Check sheet for the modelled part. Datum: model origin and axes. Units: mm. Face numbers are marked on the shaded views. A direction names the side the tool comes from. Round coordinates to 2 decimals unless told otherwise and drop trailing zeros. Loops run counter-clockwise (first coordinate to the right, second up) from the corner with the lowest first, then second, coordinate; pieces in that order, holes last. Notation, with made-up numbers: (-6, 12) -> (36, 12) arc R31 cw to (36, 46) -> close; hole circle Ø5 at (6.5, -13). An arc over 180 degrees is marked (long way). One line per question, with ' | ' between items.
```python
from build123d import *

# Parameters (mm, degrees)
F1_DEPTH = 5
F2_W     = 5
F2_H     = 5
F3_DEPTH = 12
F4_R     = 1.5
F5_DEPTH = 20


with BuildPart() as f1:
    # F0 (on Right) → F1 (new body, symmetric)
    with BuildSketch(Plane.YZ):
        Polygon((-5.680779, 3.206832), (-10.680779, 3.206832), (-20.680779, -6.793168), (-5.680779, -6.793168), align=None)
    extrude(amount=F1_DEPTH, both=True)

    # F2 (on face) → F3 (join)
    with BuildSketch(Plane.XY.offset(3.206832)):
        with Locations((2.5, -8.180779)):
            Rectangle(F2_W, F2_H)
    extrude(amount=F3_DEPTH)

    # F4 (on face) → F5 (join)
    with BuildSketch(Plane.XY.offset(3.206832)):
        with Locations((-2.5, -8.180779)):
            Circle(F4_R)
    extrude(amount=F5_DEPTH)


solid = f1.part
```
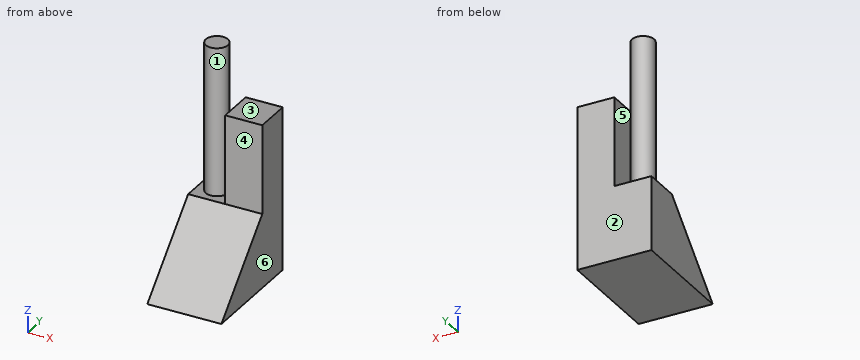
(1) Sectioned sample at A-A, the plane x = -2.75. Record the cut outline in (y, z).
Answer:
outline: (-20.68, -6.79) -> (-5.68, -6.79) -> (-5.68, 3.21) -> (-6.7, 3.21) -> (-6.7, 23.21) -> (-9.66, 23.21) -> (-9.66, 3.21) -> (-10.68, 3.21) -> close
(2) Go/stop test with flat-tipped pins: pin 1 (5.5 mm diameter, centred on x = 1.5, y = -7.5, fed in from +Z); pin 2 (1 mm diameter, centred on x = -2, y = -17, fed in from +Z); pin 3 (1.5 mm diameter, centred on x = 1.5, z = 7.5, fed in from -Y); pin 4 (6 mm diameter, centred on y = -12, z = 13, fed in from -X). Record where each tip stops, or that it passes through.
Answer:
pin 1: stops at z = 23.21 | pin 2: stops at z = -2.61 | pin 3: stops at y = -10.68 | pin 4: stops at x = -3.76
(3) Sectioned sample at D-D, the plane z = -1.5. Record the cut outline in (x, y), and give its area (3 significant figures).
Answer:
outline: (-5, -15.39) -> (5, -15.39) -> (5, -5.68) -> (-5, -5.68) -> close | area: 97.1 mm2
(4) Mould release check, pull along X, two halves, no side actions. Record for the marked faces 4, 5 and 6: +X half, -X half, draft (parallel to the pull), parting line (faces both ways), or undercut.
Answer:
face 4: draft | face 5: undercut | face 6: +X half
(5) Set-up check for the marked faces 1, 2 and 3: record each of +Z, -Z, +X, -X, +Y, -Y from which the full face is reachable in a straight line by a thin tool's end or side.
Answer:
face 1: +Z | face 2: +Z, -Z, +X, -X, +Y | face 3: +Z, +X, +Y, -Y
(6) Sectioned sample at B-B, the plane z = 7. Record the cut outline in (x, y), and give its area (3 significant figures).
Answer:
outline: circle Ø3 at (-2.5, -8.18); (0, -10.68) -> (5, -10.68) -> (5, -5.68) -> (0, -5.68) -> close | area: 32.1 mm2
(7) Sectioned sample at C-C, the plane y = -7.5. Record the cut outline in (x, z).
Answer:
outline: (-5, -6.79) -> (5, -6.79) -> (5, 15.21) -> (0, 15.21) -> (0, 3.21) -> (-1.16, 3.21) -> (-1.16, 23.21) -> (-3.84, 23.21) -> (-3.84, 3.21) -> (-5, 3.21) -> close
(8) Scan lines: probe 1 along Y at (x, z) = (-2.5, 7.25); probe 2 along Z at (x, y) = (2.25, -8); probe 3 along X at (y, z) = (-10.5, 13.5). Record each from-to range of solid material in increasing order.
Answer:
probe 1: y = -9.68 to -6.68 | probe 2: z = -6.79 to 15.21 | probe 3: x = 0 to 5
